Part model, mm, in its own coordinate system. A direction names the side the tool comes from. Coordinates: 2 decimals unless noted, no trailing zeros. Loops run counter-clockwise (first coordinate to the right, second up) from the corner with the lowest first, then second, coordinate; pieces in that order, holes last. Notation, with made-up numbers: (2.25, 39) - (12.25, 39) arc R9 ccw to (12.25, 43) - close; hole circle Ø3 at (-5.75, 32). An arc over 180 degrees is marked (long way). Use a Markdown table: item, result. Add a question column.
1. Band-saw the part on B-B, the plane y = -54.5. Give the cut face in (x, z).
2. Band-saw the part on A-A, the plane x = -48.5. Give the cut face in (y, z), plus the area to 3 significant figures.
3. Drop a flat-ended pin along its axis: pin 1 (1.8 mm diameter, centred on x = 70.5, z = 4.5, fed in from +Y). Give the stop position or say it passes through.
4. Pull direction X, two halves, no side cores. Call faces 5 (the flat face through (93.5, 3, 3)), 6 (the flat face through (-60, -66, 3)), 7 (the flat face through (0, 0, 3)), 8 (the flat face through (6, 3, 3)): pulls with the +X half, pulls with the -X half, needs draft (parallel to the pull), parting line crosses it, or undercut.
5. 3-axis set-ups, long thin cutter, end or side, ignore diameter. For faces 1 (the flat face through (90, -24, 3)), 2 (the flat face through (30, 3, 3)), 3 (the flat face through (-30, -63, 3)), 4 (the flat face through (-91, -48, 3)): which of +Z, -Z, +X, -X, +Y, -Y reach the whole face in a straight line?
6. Wall check: probe 1 along Y at (x, z) = (29, 1.1); probe 2 along X at (y, z) = (-29, 4.05). Give the ranges that are in metal, low to high. Write a range as [from, to].
from build123d import *

# Parameters (mm, degrees)
SKETCH1_W           = 6
SKETCH1_H           = 12
BOSS_EXTRUDE3_DEPTH = 6
SKETCH3_W           = 6
SKETCH3_H           = 12
CUT_EXTRUDE1_DEPTH  = 6
SKETCH4_W           = 12
SKETCH4_H           = 6
CUT_EXTRUDE2_DEPTH  = 6


with BuildPart() as part:
    # Sketch1 → Boss-Extrude3 (new body)
    with BuildSketch(Plane.XY):
        Polygon((-93.5, 6), (-93.5, -66), (93.5, -66), (93.5, 6), (78, 6), (78, 0), (66, 0), (66, 6), (54, 6), (54, 0), (42, 0), (42, 6), (30, 6), (30, 0), (18, 0), (18, 6), (6, 6), (6, 0), (-6, 0), (-6, 6), (-18, 6), (-18, 0), (-30, 0), (-30, 6), (-42, 6), (-42, 0), (-54, 0), (-54, 6), (-66, 6), (-66, 0), (-78, 0), (-78, 6), align=None)
        with Locations((90.5, -6)):
            Rectangle(SKETCH1_W, SKETCH1_H)
        with Locations((90.5, -30)):
            Rectangle(SKETCH1_W, SKETCH1_H)
        with Locations((90.5, -54)):
            Rectangle(SKETCH1_W, SKETCH1_H)
    extrude(amount=BOSS_EXTRUDE3_DEPTH)

    # Sketch3 → Cut-Extrude1 (cut)
    with BuildSketch(Plane.XY.offset(6)):
        with Locations((-90.5, -6)):
            Rectangle(SKETCH3_W, SKETCH3_H)
        with Locations((90.5, -6)):
            Rectangle(SKETCH3_W, SKETCH3_H)
        with Locations((90.5, -30)):
            Rectangle(SKETCH3_W, SKETCH3_H)
        with Locations((90.5, -54)):
            Rectangle(SKETCH3_W, SKETCH3_H)
        with Locations((-90.5, -30)):
            Rectangle(SKETCH3_W, SKETCH3_H)
        with Locations((-90.5, -54)):
            Rectangle(SKETCH3_W, SKETCH3_H)
    extrude(amount=-CUT_EXTRUDE1_DEPTH, mode=Mode.SUBTRACT)

    # Sketch4 → Cut-Extrude2 (cut)
    with BuildSketch(Plane.XY.offset(6)):
        with Locations((-72, -63)):
            Rectangle(SKETCH4_W, SKETCH4_H)
        with Locations((-48, -63)):
            Rectangle(SKETCH4_W, SKETCH4_H)
        with Locations((-24, -63)):
            Rectangle(SKETCH4_W, SKETCH4_H)
        with Locations((0, -63)):
            Rectangle(SKETCH4_W, SKETCH4_H)
        with Locations((24, -63)):
            Rectangle(SKETCH4_W, SKETCH4_H)
        with Locations((48, -63)):
            Rectangle(SKETCH4_W, SKETCH4_H)
        with Locations((72, -63)):
            Rectangle(SKETCH4_W, SKETCH4_H)
    extrude(amount=-CUT_EXTRUDE2_DEPTH, mode=Mode.SUBTRACT)


solid = part.part
Geometry check:
| question | item | result |
|---|---|---|
| 1 | outline | (-87.5, 0) - (87.5, 0) - (87.5, 6) - (-87.5, 6) - close |
| 2 | outline | (-60, 0) - (0, 0) - (0, 6) - (-60, 6) - close |
| 2 | area | 360 mm^2 |
| 3 | pin 1 | stops at y = 0 |
| 4 | face 5 | pulls with the +X half |
| 4 | face 6 | needs draft |
| 4 | face 7 | undercut |
| 4 | face 8 | undercut |
| 5 | face 1 | +Z, -Z, +X |
| 5 | face 2 | +Z, -Z, +Y |
| 5 | face 3 | +Z, -Z, -Y |
| 5 | face 4 | +Z, -Z, -X |
| 6 | probe 1 | y = [-60, 0] |
| 6 | probe 2 | x = [-87.5, 87.5] |
